Geometry check sheet. Reference: the model listing, model coordinates, mm. A direction names the side the tool comes from. Coordinates: 2 decimals unless noted, no trailing zeros. Write each loop counter-clockwise with the first axis right and the second up, starting at its lowest first coordinate (ties: lowest second). Pieces come first, ordered by that corner, then holes. Notation, with made-up numbers: (64, 56) -> (91, 56) arc R34 ccw to (91, 93) -> close; hole circle Ø9 at (45.25, 69). An arc over 180 degrees is marked (long way). Answer in a Markdown table with one row per item. Add a question column.
Q1. Release check for a two-part mould opening along X. For faces 1 (the face through (11.5, 0, 254)), 2 (the face through (0, -12.5, 246)), 3 (the face through (12.5, 0, 246)) record: pulls with the +X half, pulls with the -X half, needs draft (parallel to the pull), parting line crosses it, or undercut.
Q2. Section check D-D, the plane z = 15. Record the boundary of the cut face in (x, y).
Q3. Gauge pin test, flat end, axial feed: P1, Ø6, axis at x = -6, y = 2.5, coming from the +Z side. Record the tip position at first contact, or that the pin passes through.
Q4. Section check C-C, the plane z = 372. Record the boundary of the cut face in (x, y).
Q5. Thickness scan on line 1 (Y direction, x = -10.75, z = 54); line 2 (Z direction, x = -12.05, y = 0). Record the ranges inside material, lowest first.
Q6. Tool access check on faces 4 (the face through (0, 11.5, 254)), 5 (the face through (-1, -12, 0)). Record the directions out of +Z, -Z, +X, -X, +Y, -Y that give a thin tool (end or side, any length) a straight path to the whole face; none if there is none.
Q7. Section check B-B, the plane y = 0. Record the boundary of the cut face in (x, z).
Q8. Section check A-A, the plane x = 0. Record the boundary of the cut face in (y, z).
```python
from build123d import *

# Parameters (mm, degrees)
SKETCH1_W           = 25
SKETCH1_H           = 25
BOSS_EXTRUDE1_DEPTH = 500
SKETCH2_W           = 23
SKETCH2_H           = 23
CUT_EXTRUDE1_DEPTH  = 501.312402405
SKETCH3_R           = 6.75
CUT_EXTRUDE2_DEPTH  = 501.7806406


with BuildPart() as part:
    # Sketch1 → Boss-Extrude1 (new body)
    with BuildSketch(Plane.XY):
        Rectangle(SKETCH1_W, SKETCH1_H)
    extrude(amount=BOSS_EXTRUDE1_DEPTH)

    # Sketch2 → Cut-Extrude1 (cut, through all)
    with BuildSketch(Plane.XY.offset(500)):
        Rectangle(SKETCH2_W, SKETCH2_H)
    extrude(amount=-CUT_EXTRUDE1_DEPTH, mode=Mode.SUBTRACT)

    # Sketch3 → Cut-Extrude2 (cut, through all)
    with BuildSketch(Plane(origin=(12.5, 0, 0), x_dir=(0, 0, -1), z_dir=(1, 0, 0))):
        with Locations(Location((-15, 0, 0), (0, 0, 90))):
            Circle(SKETCH3_R)
    extrude(amount=-CUT_EXTRUDE2_DEPTH, mode=Mode.SUBTRACT)


solid = part.part
```
Calculated:
| question | item | result |
|---|---|---|
| 1 | face 1 | undercut |
| 1 | face 2 | needs draft |
| 1 | face 3 | pulls with the +X half |
| 2 | outline | (-12.5, -12.5) -> (12.5, -12.5) -> (12.5, -6.75) -> (11.5, -6.75) -> (11.5, -11.5) -> (-11.5, -11.5) -> (-11.5, -6.75) -> (-12.5, -6.75) -> close; (-12.5, 6.75) -> (-11.5, 6.75) -> (-11.5, 11.5) -> (11.5, 11.5) -> (11.5, 6.75) -> (12.5, 6.75) -> (12.5, 12.5) -> (-12.5, 12.5) -> close |
| 3 | P1 | passes through |
| 4 | outline | (-12.5, -12.5) -> (12.5, -12.5) -> (12.5, 12.5) -> (-12.5, 12.5) -> close; hole (-11.5, -11.5) -> (11.5, -11.5) -> (11.5, 11.5) -> (-11.5, 11.5) -> close |
| 5 | line 1 | y = -12.5 to -11.5, 11.5 to 12.5 |
| 5 | line 2 | z = 0 to 8.25, 21.75 to 500 |
| 6 | face 4 | +Z, -Z |
| 6 | face 5 | -Z, +X, -X, +Y, -Y |
| 7 | outline | (-12.5, 0) -> (-11.5, 0) -> (-11.5, 8.25) -> (-12.5, 8.25) -> close; (-12.5, 21.75) -> (-11.5, 21.75) -> (-11.5, 500) -> (-12.5, 500) -> close; (11.5, 0) -> (12.5, 0) -> (12.5, 8.25) -> (11.5, 8.25) -> close; (11.5, 21.75) -> (12.5, 21.75) -> (12.5, 500) -> (11.5, 500) -> close |
| 8 | outline | (-12.5, 0) -> (-11.5, 0) -> (-11.5, 500) -> (-12.5, 500) -> close; (11.5, 0) -> (12.5, 0) -> (12.5, 500) -> (11.5, 500) -> close |
